Build history of the part. All positions in model axes, mm. A direction names the side the tool comes from. Round coordinates to 2 decimals unless told otherwise and drop trailing zeros. Order: outer loops, then holes, each group sorted by start corner. A loop starts at its lowest first (then second) coordinate and runs counter-clockwise, first axis right, second up. Notation, with made-up numbers: M -7.75,16 L 20.25,16 A31 cw 20.25,49 Z; hole C -20.75,41 d5. An arc over 180 degrees is marked long. Use CSV: the item, a comma, the result in double quotes.
from build123d import *

# Parameters (mm, degrees)
SKETCH1_W           = 113
SKETCH1_H           = 166
BOSS_EXTRUDE1_DEPTH = 2
CUT_EXTRUDE1_REACH  = 102.425
SKETCH2_R           = 2.5
SKETCH2_W           = 8
SKETCH2_H           = 4
FILLET1_R           = 2
SKETCH3_W           = 40
SKETCH3_H           = 5
BOSS_EXTRUDE2_DEPTH = 10
CUT_EXTRUDE2_REACH  = 116.062
SKETCH5_R           = 19
CUT_EXTRUDE3_REACH  = 116.062
SKETCH6_R           = 2
CUT_EXTRUDE4_REACH  = 103.12
SKETCH7_W           = 52.844902502
SKETCH7_H           = 42.914109563
FILLET2_R           = 2


with BuildPart() as part:
    # Sketch1 → Boss-Extrude1 (new body)
    with BuildSketch(Plane(origin=(0, 0, 0), x_dir=(1, 0, 0), z_dir=(0, 1, 0))):
        Rectangle(SKETCH1_W, SKETCH1_H)
    extrude(amount=BOSS_EXTRUDE1_DEPTH)

    # Sketch2 → Cut-Extrude1 (cut, up to next)
    with BuildSketch(Plane(origin=(0, 2, 0), x_dir=(1, 0, 0), z_dir=(0, 1, 0)), mode=Mode.PRIVATE) as cut_extrude1_sk1:
        with Locations(Location((51.5, 76, 0), (0, 0, 270))):
            Circle(SKETCH2_R)
    cut_extrude1_tool1 = extrude(cut_extrude1_sk1.sketch, amount=-CUT_EXTRUDE1_REACH, mode=Mode.PRIVATE) & part.part
    # Sketch2 → Cut-Extrude1 (cut, up to next)
    with BuildSketch(Plane(origin=(0, 2, 0), x_dir=(1, 0, 0), z_dir=(0, 1, 0)), mode=Mode.PRIVATE) as cut_extrude1_sk2:
        with Locations(Location((-50.5, 76, 0), (0, 0, 270))):
            Circle(SKETCH2_R)
    cut_extrude1_tool2 = extrude(cut_extrude1_sk2.sketch, amount=-CUT_EXTRUDE1_REACH, mode=Mode.PRIVATE) & part.part
    # Sketch2 → Cut-Extrude1 (cut, up to next)
    with BuildSketch(Plane(origin=(0, 2, 0), x_dir=(1, 0, 0), z_dir=(0, 1, 0)), mode=Mode.PRIVATE) as cut_extrude1_sk3:
        with Locations((-1.5, -53)):
            Rectangle(SKETCH2_W, SKETCH2_H)
    cut_extrude1_tool3 = extrude(cut_extrude1_sk3.sketch, amount=-CUT_EXTRUDE1_REACH, mode=Mode.PRIVATE) & part.part
    add(cut_extrude1_tool1.solids().sort_by_distance((51.5, 2, -76))[0], mode=Mode.SUBTRACT)
    add(cut_extrude1_tool2.solids().sort_by_distance((-50.5, 2, -76))[0], mode=Mode.SUBTRACT)
    add(cut_extrude1_tool3.solids().sort_by_distance((-1.5, 2, 53))[0], mode=Mode.SUBTRACT)

    # Fillet1
    fillet1_edges = [part.edges().sort_by_distance(p)[0] for p in [
        (-5.5, 1, 55),
        (-5.5, 1, 51),
        (2.5, 1, 55),
        (2.5, 1, 51),
    ]]
    fillet(fillet1_edges, radius=FILLET1_R - 0.0001)  # a hair under: the kernel refuses the full size

    # Sketch3 → Boss-Extrude2 (add)
    with BuildSketch(Plane.XZ):
        with Locations((-8.5, 13.079652709)):
            Rectangle(SKETCH3_W, SKETCH3_H)
    extrude(amount=BOSS_EXTRUDE2_DEPTH)

    # Sketch5 → Cut-Extrude2 (cut, up to next)
    with BuildSketch(Plane.XY.offset(15.579652709), mode=Mode.PRIVATE) as cut_extrude2_sk1:
        with Locations((-8.538915201, -19)):
            Circle(SKETCH5_R)
    cut_extrude2_tool1 = extrude(cut_extrude2_sk1.sketch, amount=-CUT_EXTRUDE2_REACH, mode=Mode.PRIVATE) & part.part
    add(cut_extrude2_tool1.solids().sort_by_distance((-8.538915, -19, 15.579653))[0], mode=Mode.SUBTRACT)

    # Sketch6 → Cut-Extrude3 (cut, up to next)
    with BuildSketch(Plane.XY.offset(15.579652709), mode=Mode.PRIVATE) as cut_extrude3_sk1:
        with Locations((7.5, -4)):
            Circle(SKETCH6_R)
    cut_extrude3_tool1 = extrude(cut_extrude3_sk1.sketch, amount=-CUT_EXTRUDE3_REACH, mode=Mode.PRIVATE) & part.part
    cut_extrude3 = cut_extrude3_tool1.solids().sort_by_distance((7.5, -4, 15.579653))[0]
    add(cut_extrude3, mode=Mode.SUBTRACT)

    # Mirror1: Cut-Extrude3 across plane
    add(cut_extrude3.mirror(Plane(origin=(-8.5, 0, 0), x_dir=(0, 0, 1), z_dir=(1, 0, 0))), mode=Mode.SUBTRACT)

    # Sketch7 → Cut-Extrude4 (cut, up to next)
    with BuildSketch(Plane(origin=(0, 2, 0), x_dir=(1, 0, 0), z_dir=(0, 1, 0)), mode=Mode.PRIVATE) as cut_extrude4_sk1:
        with Locations((2.514142356, 46.957054782)):
            Rectangle(SKETCH7_W, SKETCH7_H)
    cut_extrude4_tool1 = extrude(cut_extrude4_sk1.sketch, amount=-CUT_EXTRUDE4_REACH, mode=Mode.PRIVATE) & part.part
    add(cut_extrude4_tool1.solids().sort_by_distance((2.514142, 2, -46.957055))[0], mode=Mode.SUBTRACT)

    # Fillet2
    fillet2_edges = [part.edges().sort_by_distance(p)[0] for p in [
        (28.936593607, 1, -68.414109563),
        (28.936593607, 1, -25.5),
        (-23.908308895, 1, -25.5),
        (-23.908308895, 1, -68.414109563),
    ]]
    fillet(fillet2_edges, radius=FILLET2_R)


solid = part.part
(1) Tool access for faces 1 (the face through (5.502, -3.912, 13.115)), 2 (the face through (-22, -3, 10.58)), 3 (the face through (5, -4, 15.58)): list every direction of +Z, -Z, +X, -X, +Y, -Y with a clear straight run to the whole face (end or side of a thin tool).
Answer block:
face 1,"+Z, -Z"
face 2,"-Z, +X, -X, -Y"
face 3,"+Z, +X, -X, -Y"
(2) Cut at D-D, the plane x = -31. Give the cut face in (y, z), and give its area (3 significant figures).
Answer block:
outline,"M 0,-83 L 2,-83 L 2,83 L 0,83 Z"
area,"332 mm²"
(3) Cut at A-A, the plane x = -50.5. Give the cut face in (y, z).
Answer block:
outline,"M 0,-83 L 2,-83 L 2,-78.5 L 0,-78.5 Z; M 0,-73.5 L 2,-73.5 L 2,83 L 0,83 Z"
(4) Wall check: line 1 (X direction, y = 1.4, z = -76); line 2 (Y direction, x = -44.5, z = -25.5); line 3 (Y direction, x = -24, z = 13). Give the ranges that are in metal, low to high. Write a range as from..to.
Answer block:
line 1,"x = -56.5..-53, -48..49, 54..56.5"
line 2,"y = 0..2"
line 3,"y = -7.96..-5.94, -2.06..2"
(5) Cut at B-B, the plane z = -42.5. Give the cut face in (x, y), and give its area (3 significant figures).
Answer block:
outline,"M -56.5,0 L -23.91,0 L -23.91,2 L -56.5,2 Z; M 28.94,0 L 56.5,0 L 56.5,2 L 28.94,2 Z"
area,"120 mm²"
(6) Drop flat-ended pins along their axis: pin 1 (1.5 mm diameter, centred on x = -43, z = 14, fed in from -Y); pin 2 (5.5 mm diameter, centred on y = -3, z = 13, fed in from -X); pin 3 (5.5 mm diameter, centred on y = -6, z = 14, fed in from +X). Give the stop position or say it passes through.
Answer block:
pin 1,"stops at y = 0"
pin 2,"stops at x = -28.5"
pin 3,"stops at x = 11.5"
(7) Cut at C-C, the plane z = 13. Give the cut face in (x, y), and give its area (3 significant figures).
Answer block:
outline,"M -56.5,0 L -28.5,0 L -28.5,-10 L -25.27,-10 A19 cw 8.19,-10 L 11.5,-10 L 11.5,0 L 56.5,0 L 56.5,2 L -56.5,2 Z; hole C -24.5,-4 d4; hole C 7.5,-4 d4"
area,"363 mm²"
(8) Two-plate mould, pull along X, no slides. Class faces 4 (the face through (-28.5, -5, 13)), 5 (the face through (11.5, -5, 13)), 6 (the face through (-22.502, -3.912, 13.115)): released by +X, released by -X, zero draft, split by the parting line, or undercut.
Answer block:
face 4,"released by -X"
face 5,"released by +X"
face 6,"undercut"
